```python
from build123d import *

# Parameters (mm, degrees)
SZKIC1_W                    = 100
SZKIC1_H                    = 100
DODANIE_WYCI_GNI_CIE1_DEPTH = 4
DODANIE_WYCI_GNI_CIE3_DEPTH = 196


with BuildPart() as part:
    # Szkic1 → Dodanie-wyciągnięcie1 (new body)
    with BuildSketch(Plane.XY):
        with Locations((-50, 50)):
            Rectangle(SZKIC1_W, SZKIC1_H)
        with Locations((50, 50)):
            Rectangle(SZKIC1_W, SZKIC1_H)
        with Locations((50, -50)):
            Rectangle(SZKIC1_W, SZKIC1_H)
        with Locations((-50, -50)):
            Rectangle(SZKIC1_W, SZKIC1_H)
    extrude(amount=DODANIE_WYCI_GNI_CIE1_DEPTH)

    # Szkic2 → Dodanie-wyciągnięcie3 (add)
    with BuildSketch(Plane.XY.offset(4)):
        Polygon((100, 3), (3, 3), (3, 100), (-3, 100), (-3, -3), (100, -3), align=None)
    extrude(amount=DODANIE_WYCI_GNI_CIE3_DEPTH)


solid = part.part
```
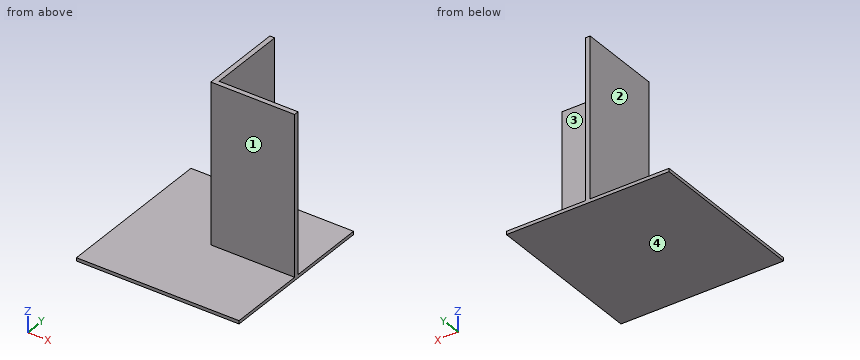
Verification items for the finished model (mm, model axes). Face numbers are marked on the shaded views. A direction names the side the tool comes from. Coordinates: 2 decimals unless noted, no trailing zeros. Order: outer loops, then holes, each group sorted by start corner. A loop starts at its lowest first (then second) coordinate and runs counter-clockwise, first axis right, second up. Notation, with made-up numbers: (67.5, -37.5) -> (109.5, -37.5) arc R27 ccw to (109.5, 1.5) -> close; hole circle Ø6 at (9, -5). An arc over 180 degrees is marked (long way). Answer as CSV lines item,"result". Start each with the question number.
1) Cross-section at B-B, the plane z = 187.5. Record the boundary of the cut face in (x, y).
2) Cross-section at A-A, the plane x = 61. Record the boundary of the cut face in (y, z), then the cut area to 3 significant figures.
3) Cross-section at C-C, the plane y = -60. Record the boundary of the cut face in (x, z).
4) Set-up check for the marked faces 1, 2, 3 and 4: record each of +Z, -Z, +X, -X, +Y, -Y from which the full face is reachable in a straight line by a thin tool's end or side.
5) Cross-section at D-D, the plane x = 0. Record the boundary of the cut face in (y, z).
6) Gauge pin test, flat ends, axial feed: pin 1 Ø5 at (y, z) = (23, 80.5) entering from -X; pin 2 Ø10 at (y, z) = (67.5, 54) entering from +X; pin 3 Ø8 at (x, y) = (-53, -19.5) entering from +Z. Record the tip position at first contact, or that the pin passes through.
7) Material ranges on L1, parallel to Z at x = -75, y = 13.5; L2, parallel to Y at x = 55, z = 79, recorded low to high. Write a range as [from, to].
Conclusion:
1,outline,"(-3, -3) -> (100, -3) -> (100, 3) -> (3, 3) -> (3, 100) -> (-3, 100) -> close"
2,outline,"(-100, 0) -> (100, 0) -> (100, 4) -> (3, 4) -> (3, 200) -> (-3, 200) -> (-3, 4) -> (-100, 4) -> close"
2,area,"1,980 mm²"
3,outline,"(-100, 0) -> (100, 0) -> (100, 4) -> (-100, 4) -> close"
4,face 1,"+Z, +X, -X, -Y"
4,face 2,"+Z, -X, +Y, -Y"
4,face 3,"+Z, +X, +Y"
4,face 4,"-Z, +X, -X, +Y, -Y"
5,outline,"(-100, 0) -> (100, 0) -> (100, 200) -> (-3, 200) -> (-3, 4) -> (-100, 4) -> close"
6,pin 1,"stops at x = -3"
6,pin 2,"stops at x = 3"
6,pin 3,"stops at z = 4"
7,L1,"z = [0, 4]"
7,L2,"y = [-3, 3]"
